from build123d import *

# Parameters (mm, degrees)
BOSS_EXTRUDE1_DEPTH      = 74.93
BOSS_EXTRUDE4_DEPTH      = 2.54
BOSS_EXTRUDE4_DEPTH_BACK = 2.54
BOSS_EXTRUDE6_DEPTH      = 74.93
BOSS_EXTRUDE7_DEPTH      = 74.93
SKETCH11_R               = 3.3782
BOSS_EXTRUDE8_DEPTH      = 2.54
SKETCH12_R               = 3.175
BOSS_EXTRUDE9_DEPTH      = 11.43
SKETCH14_W               = 11.454369962
SKETCH14_H               = 4.541337636
BOSS_EXTRUDE10_DEPTH     = 5.08
SKETCH16_R               = 4.043569484
BOSS_EXTRUDE11_DEPTH     = 5.08


with BuildPart() as part:
    # Sketch1 → Boss-Extrude1 (new body)
    with BuildSketch(Plane.XY):
        with BuildLine():
            Line((-16.295773791, 0.624640473), (-12.907508233, 0.624640473))
            Line((-12.907508233, 0.624640473), (-12.443267089, 3.164640473))
            add(Edge.make_bspline(
                [(-12.443267089, 3.164640473), (-12.30668745, 3.911907895), (-11.89696139, 6.153716378), (-11.35075536, 9.142778811), (-10.941162808, 11.384616955), (-10.804635025, 12.131895145)],
                knots=[0.002076118, 0.002076118, 0.002076118, 0.002076118, 0.004355051, 0.008912916, 0.011191849, 0.011191849, 0.011191849, 0.011191849], degree=3))
            add(Edge.make_bspline(
                [(-10.804635025, 12.131895145), (-10.131787944, 14.813925559), (-8.428636773, 20.08894476), (-4.769918918, 27.602373316), (-0.882056925, 33.370017928), (2.696640916, 37.629074894), (4.663596703, 39.6688962), (5.677623009, 40.647244333)],
                knots=[-0.595137067, -0.595137067, -0.595137067, -0.595137067, -0.254899084, 0.0853389, 0.425576884, 0.595695875, 0.765814867, 0.765814867, 0.765814867, 0.765814867], degree=3))
            Line((5.677623009, 40.647244333), (2.03170084, 44.371046934))
            add(Edge.make_bspline(
                [(2.03170084, 44.371046934), (1.545061943, 43.849333503), (0.584048879, 42.784657511), (-1.227882281, 40.634272171), (-4.205920413, 36.737641226), (-7.868630072, 30.842728735), (-11.285075765, 23.259160615), (-12.891126954, 17.928422411), (-13.516382283, 15.22778531)],
                knots=[0.192222826, 0.192222826, 0.192222826, 0.192222826, 0.287167093, 0.38211136, 0.571999893, 0.951776961, 1.331554028, 1.711331096, 1.711331096, 1.711331096, 1.711331096], degree=3))
            add(Edge.make_bspline(
                [(-13.516382283, 15.22778531), (-13.707651088, 14.222513225), (-14.09021448, 12.211975656), (-14.664139503, 9.196174334), (-15.238140346, 6.180406911), (-15.620861993, 4.169893716), (-15.812232602, 3.164640473)],
                knots=[-0.00268258, -0.00268258, -0.00268258, -0.00268258, 0.000387339, 0.003457258, 0.006527177, 0.009597097, 0.009597097, 0.009597097, 0.009597097], degree=3))
            Line((-15.812232602, 3.164640473), (-16.295773791, 0.624640473))
        make_face()
    extrude(amount=BOSS_EXTRUDE1_DEPTH)

    # Sketch4 → Boss-Extrude4 (add, two sides: drawn at the far end of the back side and taken through both)
    with BuildSketch(Plane(origin=(0, 0, 37.465), x_dir=(-1, 0, 0), z_dir=(0, 0, -1)).offset(-BOSS_EXTRUDE4_DEPTH_BACK)):
        with BuildLine():
            Line((-5.677623009, 40.647244333), (-2.087143894, 44.314419562))
            ThreePointArc((-2.087143894, 44.314419562), (-5.945357936, 46.761917563), (-10.144870483, 48.561961011))
            Line((-10.144870483, 48.561961011), (-12.342217859, 43.933321468))
            ThreePointArc((-12.342217859, 43.933321468), (-8.878894593, 42.556020468), (-5.677623009, 40.647244333))
        make_face()
    extrude(amount=BOSS_EXTRUDE4_DEPTH + BOSS_EXTRUDE4_DEPTH_BACK)

    # Sketch8 → Boss-Extrude6 (add)
    with BuildSketch(Plane(origin=(0, 0, 0), x_dir=(-1, 0, 0), z_dir=(0, 0, -1))):
        with BuildLine():
            Line((12.199993526, 0.628671187), (16.843743367, 0.628671187))
            add(Edge.make_bspline(
                [(-2.03170084, 44.371046934), (15.008940659, 25.494574417), (16.843743367, 0.628671187)],
                knots=[0, 0, 0, 1, 1, 1], degree=2))
            Line((-2.03170084, 44.371046934), (-5.677623009, 40.647244333))
            add(Edge.make_bspline(
                [(-5.677623009, 40.647244333), (9.879032096, 23.52153238), (12.199993526, 0.628671187)],
                knots=[0, 0, 0, 1, 1, 1], degree=2))
        make_face()
    extrude(amount=-BOSS_EXTRUDE6_DEPTH)

    # Sketch10 → Boss-Extrude7 (add)
    with BuildSketch(Plane.XY.offset(74.93)):
        with BuildLine():
            add(Edge.make_bspline(
                [(-17.044210577, -3.569022053), (-16.99706974, -1.449262713), (-16.843743367, 0.628671187)],
                knots=[0, 0, 0, 1, 1, 1], degree=2))
            Line((-16.843743367, 0.628671187), (-16.295006462, 0.628671187))
            Line((-16.295006462, 0.628671187), (-16.295773791, 0.624640473))
            Line((-16.295773791, 0.624640473), (-12.907508233, 0.624640473))
            Line((-12.907508233, 0.624640473), (-12.906771531, 0.628671187))
            Line((-12.906771531, 0.628671187), (-12.199993526, 0.628671187))
            add(Edge.make_bspline(
                [(-12.199993526, 0.628671187), (-12.410380076, -1.44648182), (-12.512012235, -3.569022053)],
                knots=[0, 0, 0, 1, 1, 1], degree=2))
            Line((-12.512012235, -3.569022053), (-17.044210577, -3.569022053))
        make_face()
    extrude(amount=-BOSS_EXTRUDE7_DEPTH)

    # Sketch11 → Boss-Extrude8 (add, symmetric)
    with BuildSketch(Plane(origin=(0, 0, 37.465), x_dir=(-1, 0, 0), z_dir=(0, 0, -1))):
        with BuildLine():
            Line((-6.661648357, 45.739913105), (-10.144870483, 48.561961011))
            Line((-10.144870483, 48.561961011), (-21.306209309, 34.387494774))
            ThreePointArc((-21.306209309, 34.387494774), (-21.997885217, 32.978248014), (-22.052439991, 31.409358033))
            add(Edge.make_bspline(
                [(-43.921175132, 3.682891736), (-14.804010115, 3.685410597), (-22.052439991, 31.409358033)],
                knots=[0, 0, 0, 1, 1, 1], degree=2))
            ThreePointArc((-43.921175132, 3.682891736), (-45.412252296, 3.255494908), (-46.603036961, 2.261507464))
            Line((-46.603036961, 2.261507464), (-49.3060524, -1.171217021))
            ThreePointArc((-49.3060524, -1.171217021), (-49.803661042, -1.091013739), (-50.306976812, -1.06417788))
            Line((-50.306976812, -1.06417788), (-53.763973591, 15.454073405))
            ThreePointArc((-53.763973591, 15.454073405), (-56.832870033, 17.694796121), (-59.377686579, 14.872939923))
            Line((-59.377686579, 14.872939923), (-54.315487208, -3.280299501))
            ThreePointArc((-54.315487208, -3.280299501), (-50.756874344, -10.509444763), (-45.894543202, -4.084337558))
            Line((-45.894543202, -4.084337558), (-43.766648862, -1.381994502))
            ThreePointArc((-43.766648862, -1.381994502), (-42.486290668, -0.41252926), (-40.895291759, -0.193663017))
            ThreePointArc((-40.895291759, -0.193663017), (-20.913927056, 8.075766362), (-17.561546975, 29.439285396))
            ThreePointArc((-17.561546975, 29.439285396), (-17.72193531, 31.037238944), (-17.079804086, 32.509260496))
            Line((-17.079804086, 32.509260496), (-11.95129503, 39.022267547))
            Line((-11.95129503, 39.022267547), (-6.661648357, 45.739913105))
        make_face()
        with Locations((-50.306976812, -5.797526095)):
            Circle(SKETCH11_R, mode=Mode.SUBTRACT)
    extrude(amount=BOSS_EXTRUDE8_DEPTH, both=True)

    # Sketch12 → Boss-Extrude9 (add)
    with BuildSketch(Plane.XY.offset(40.005)):
        with Locations((56.540750517, 14.872939923)):
            Circle(SKETCH12_R)
    extrude(amount=-BOSS_EXTRUDE9_DEPTH)


with BuildPart() as body_2:
    # Split1: the piece on the far side of the plane
    add(part.part)
    split(bisect_by=Plane(origin=(24.222018339, -9.793178229, 0), x_dir=(-0.37483189290442787, -0.9270927958201831, 0), z_dir=(-0.9270927958201831, 0.37483189290442787, 0)), keep=Keep.BOTTOM)


with BuildPart() as part_1:
    add(part.part)

    # Split1
    split(bisect_by=Plane(origin=(24.222018339, -9.793178229, 0), x_dir=(-0.37483189290442787, -0.9270927958201831, 0), z_dir=(-0.9270927958201831, 0.37483189290442787, 0)), keep=Keep.TOP)



with BuildPart() as body_2_1:
    # Body-Move/Copy1: moved
    add(body_2.part.moved(Location((0, 0, -6.35))))


with BuildPart() as part_2:
    add(part_1.part)

    add(body_2_1.part)  # Boss-Extrude10 merges body 2
    # Sketch14 → Boss-Extrude10 (add)
    with BuildSketch(Plane(origin=(24.222018339, -9.793178229, 0), x_dir=(0, 0, -1), z_dir=(0.9270927958201831, -0.37483189290442787, 0))):
        with Locations((-34.301669156, 14.639573878)):
            Rectangle(SKETCH14_W, SKETCH14_H)
    extrude(amount=BOSS_EXTRUDE10_DEPTH)

    # Sketch16 → Boss-Extrude11 (add)
    with BuildSketch(Plane(origin=(0, 0, 28.575), x_dir=(-1, 0, 0), z_dir=(0, 0, -1))):
        with Locations((-56.540750517, 14.872939923)):
            Circle(SKETCH16_R)
    extrude(amount=-BOSS_EXTRUDE11_DEPTH)


solid = part_2.part
Geometry: final body of the model. Coordinates: model frame, mm. A direction names the side the tool comes from. Coordinates: 2 decimals unless noted, no trailing zeros. Order: outer loops, then holes, each group sorted by start corner. A loop starts at its lowest first (then second) coordinate and runs counter-clockwise, first axis right, second up.
(1) Draft query along Y for faces 5 (the face through (17.91, 13.17, 37.43)), 6 (the face through (15.65, 41.57, 37.43)), 7 (the face through (52, 4, 33.655)), 8 (the face through (34.43, 1.9, 36.93)). Return one class per face: pulls with the +Y half, pulls with the -Y half, needs draft (parallel to the pull), parting line crosses it, or undercut.
(2) First-contact query: pin 1 (3 mm diameter, centred on y = 3.5, z = 10.5, fed in from +X); pin 2 (8.5 mm diameter, centred on x = 19, y = 32.5, fed in from +Z) (3 decimals); pin 3 (14 mm diameter, centred on x = 15.5, y = 28.5, fed in from -Z) (3 decimals). Flat tips, straight axial feed; report the tip coordinate or a pass-through.
(3) Section query A-A (y = -7). Return the cut outline in (x, z) (3 decimals).
(4) Material intervals for probe 1 along X at (y, z) = (13.5, 39.5); probe 2 along Z at (x, y) = (55, 16.5) (3 decimals); probe 3 along X at (y, z) = (0.5, 3), sorted ascending.
(5) Access query for faces 1 (the face through (54.2, 17.02, 25.44)), 2 (the face through (31.18, 0.735, 34.382)), 3 (the face through (-8, 22, 74.93)), 4 (the face through (56, 15, 22.225)). Directions: +Z, -Z, +X, -X, +Y, -Y. A direction counts if a zero-diameter tool reaches every point of the face in a straight line with its end or side. Return the directions, or none.
Solution:
1. face 5: undercut
1. face 6: pulls with the +Y half
1. face 7: needs draft
1. face 8: pulls with the -Y half
2. pin 1: stops at x = -11.63
2. pin 2: stops at z = 40.005
2. pin 3: stops at z = 34.925
3. outline: (45.729, 28.575) - (47.15, 28.575) - (47.15, 33.655) - (45.729, 33.655) - close; (53.464, 28.575) - (54.885, 28.575) - (54.885, 33.655) - (53.464, 33.655) - close
4. probe 1: x = -14.77 to -9.72, 17.77 to 22.15
4. probe 2: z = 22.225 to 33.655
4. probe 3: x = -16.85 to -12.21
5. face 1: -Z
5. face 2: +Z, -Z, -Y
5. face 3: +Z, +X, -X, +Y, -Y
5. face 4: -Z, +X, +Y, -Y
